```python
from build123d import *

# Parameters (mm, degrees)
SKETCH1_R             = 95
BOSS_EXTRUDE1_DEPTH   = 6
SKETCH2_W             = 55
SKETCH2_H             = 30
CUT_EXTRUDE1_DEPTH    = 135.484199815
CAVITY1_START         = -69.821849164
CAVITY1_OUTLINE_W     = 15
CAVITY1_OUTLINE_H     = 6
CAVITY1_OUTLINE_W_2   = 11
CAVITY1_DEPTH         = 6
CAVITY1_START_2       = 63.821772898
CAVITY1_2_OUTLINE_W   = 11
CAVITY1_2_OUTLINE_H   = 6
CAVITY1_2_OUTLINE_W_2 = 15
CAVITY1_2_DEPTH       = 6
CAVITY1_START_3       = -7.051829773
CAVITY1_3_OUTLINE_W   = 6
CAVITY1_3_OUTLINE_H   = 6
CAVITY1_3_DEPTH       = 14.103659546
CAVITY1_START_4       = -35.551829773
CAVITY1_4_OUTLINE_W   = 6
CAVITY1_4_OUTLINE_H   = 6
CAVITY1_4_DEPTH       = 10.103659546
CAVITY1_START_5       = 25.448170227
CAVITY1_5_OUTLINE_W   = 6
CAVITY1_5_OUTLINE_H   = 6
CAVITY1_5_DEPTH       = 10.103659546
CAVITY1_START_6       = -36.448170227
CAVITY1_6_OUTLINE_W   = 6
CAVITY1_6_OUTLINE_H   = 6
CAVITY1_6_DEPTH       = 0.896340454
CAVITY1_START_7       = -25.448170227
CAVITY1_7_OUTLINE_W   = 6
CAVITY1_7_OUTLINE_H   = 6
CAVITY1_7_DEPTH       = 0.896340454
CAVITY1_START_8       = -7.948170227
CAVITY1_8_OUTLINE_W   = 6
CAVITY1_8_OUTLINE_H   = 6
CAVITY1_8_DEPTH       = 0.896340454
CAVITY1_START_9       = 7.051829773
CAVITY1_9_OUTLINE_W   = 6
CAVITY1_9_OUTLINE_H   = 6
CAVITY1_9_DEPTH       = 0.896340454
CAVITY1_START_10      = 24.551829773
CAVITY1_10_OUTLINE_W  = 6
CAVITY1_10_OUTLINE_H  = 6
CAVITY1_10_DEPTH      = 0.896340454
CAVITY1_START_11      = 35.551829773
CAVITY1_11_OUTLINE_W  = 6
CAVITY1_11_OUTLINE_H  = 6
CAVITY1_11_DEPTH      = 0.896340454
SKETCH3_R             = 1.5
CUT_EXTRUDE3_DEPTH    = 10
CUT_EXTRUDE4_DEPTH    = 135.484199815
CAVITY2_START         = 73.692998072
CAVITY2_OUTLINE_W     = 6
CAVITY2_OUTLINE_H     = 6
CAVITY2_DEPTH         = 6
CUT_EXTRUDE5_DEPTH    = 135.484199815


# Read off the part's stored shape, not the designer's step: Cavity1, Cavity2
with BuildPart() as part:
    # Sketch1 → Boss-Extrude1 (new body)
    with BuildSketch(Plane(origin=(0, 0, 0), x_dir=(1, 0, 0), z_dir=(0, 1, 0))):
        with Locations(Location((0, 0, 0), (0, 0, 270))):
            Circle(SKETCH1_R)
        with BuildLine():
            Line((-36.657195747, -47.5), (36.657195747, -47.5))
            ThreePointArc((36.657195747, -47.5), (0, -60), (-36.657195747, -47.5))
        make_face(mode=Mode.SUBTRACT)
        with BuildLine():
            Line((-42.5, 42.352685865), (-42.5, -42.352685865))
            ThreePointArc((-42.5, -42.352685865), (-60, 0), (-42.5, 42.352685865))
        make_face(mode=Mode.SUBTRACT)
        with BuildLine():
            Line((36.657195747, 47.5), (-36.657195747, 47.5))
            ThreePointArc((-36.657195747, 47.5), (0, 60), (36.657195747, 47.5))
        make_face(mode=Mode.SUBTRACT)
        with BuildLine():
            Line((42.5, -42.352685865), (42.5, 42.352685865))
            ThreePointArc((42.5, 42.352685865), (60, 0), (42.5, -42.352685865))
        make_face(mode=Mode.SUBTRACT)
    extrude(amount=BOSS_EXTRUDE1_DEPTH)

    # Sketch2 → Cut-Extrude1 (cut, through all)
    with BuildSketch(Plane(origin=(0, 6, 0), x_dir=(1, 0, 0), z_dir=(0, 1, 0))):
        Rectangle(SKETCH2_W, SKETCH2_H)
    extrude(amount=-CUT_EXTRUDE1_DEPTH, mode=Mode.SUBTRACT)

    # Cavity1 outline → Cavity1 (cut)
    with BuildSketch(Plane(origin=(0, 0, 0), x_dir=(0.9999872892756082, 0, 0.005041952719030872), z_dir=(0.005041952719030872, 0, -0.9999872892756083)).offset(CAVITY1_START)):
        with Locations((0.448170227, -3)):
            Rectangle(CAVITY1_OUTLINE_W, CAVITY1_OUTLINE_H)
        with Locations((30.948170227, -3)):
            Rectangle(CAVITY1_OUTLINE_W_2, CAVITY1_OUTLINE_H)
        with Locations((-30.051829773, -3)):
            Rectangle(CAVITY1_OUTLINE_W_2, CAVITY1_OUTLINE_H)
    extrude(amount=CAVITY1_DEPTH, mode=Mode.SUBTRACT)

    # Cavity1 2 outline → Cavity1 2 (cut)
    with BuildSketch(Plane(origin=(0, 0, 0), x_dir=(0.9999872892756082, 0, 0.005041952719030872), z_dir=(0.005041952719030872, 0, -0.9999872892756083)).offset(CAVITY1_START_2)):
        with Locations((30.051829773, -3)):
            Rectangle(CAVITY1_2_OUTLINE_W, CAVITY1_2_OUTLINE_H)
        with Locations((-0.448170227, -3)):
            Rectangle(CAVITY1_2_OUTLINE_W_2, CAVITY1_2_OUTLINE_H)
        with Locations((-30.948170227, -3)):
            Rectangle(CAVITY1_2_OUTLINE_W, CAVITY1_2_OUTLINE_H)
    extrude(amount=CAVITY1_2_DEPTH, mode=Mode.SUBTRACT)

    # Cavity1 3 outline → Cavity1 3 (cut)
    with BuildSketch(Plane(origin=(0, 0, 0), x_dir=(0.9999872892756082, 0, 0.005041952719030872), z_dir=(0.005041952719030872, 0, -0.9999872892756083)).offset(CAVITY1_START_3)):
        with Locations((66.821849164, -3)):
            Rectangle(CAVITY1_3_OUTLINE_W, CAVITY1_3_OUTLINE_H)
        with Locations((-66.821849164, -3)):
            Rectangle(CAVITY1_3_OUTLINE_W, CAVITY1_3_OUTLINE_H)
    extrude(amount=CAVITY1_3_DEPTH, mode=Mode.SUBTRACT)

    # Cavity1 4 outline → Cavity1 4 (cut)
    with BuildSketch(Plane(origin=(0, 0, 0), x_dir=(0.9999872892756082, 0, 0.005041952719030872), z_dir=(0.005041952719030872, 0, -0.9999872892756083)).offset(CAVITY1_START_4)):
        with Locations((66.821849164, -3)):
            Rectangle(CAVITY1_4_OUTLINE_W, CAVITY1_4_OUTLINE_H)
        with Locations((-66.821849164, -3)):
            Rectangle(CAVITY1_4_OUTLINE_W, CAVITY1_4_OUTLINE_H)
    extrude(amount=CAVITY1_4_DEPTH, mode=Mode.SUBTRACT)

    # Cavity1 5 outline → Cavity1 5 (cut)
    with BuildSketch(Plane(origin=(0, 0, 0), x_dir=(0.9999872892756082, 0, 0.005041952719030872), z_dir=(0.005041952719030872, 0, -0.9999872892756083)).offset(CAVITY1_START_5)):
        with Locations((66.821849164, -3)):
            Rectangle(CAVITY1_5_OUTLINE_W, CAVITY1_5_OUTLINE_H)
        with Locations((-66.821849164, -3)):
            Rectangle(CAVITY1_5_OUTLINE_W, CAVITY1_5_OUTLINE_H)
    extrude(amount=CAVITY1_5_DEPTH, mode=Mode.SUBTRACT)

    # Cavity1 6 outline → Cavity1 6 (cut)
    with BuildSketch(Plane(origin=(0, 0, 0), x_dir=(0.9999872892756082, 0, 0.005041952719030872), z_dir=(0.005041952719030872, 0, -0.9999872892756083)).offset(CAVITY1_START_6)):
        with Locations((-66.821849164, -3)):
            Rectangle(CAVITY1_6_OUTLINE_W, CAVITY1_6_OUTLINE_H)
    extrude(amount=CAVITY1_6_DEPTH, mode=Mode.SUBTRACT)

    # Cavity1 7 outline → Cavity1 7 (cut)
    with BuildSketch(Plane(origin=(0, 0, 0), x_dir=(0.9999872892756082, 0, 0.005041952719030872), z_dir=(0.005041952719030872, 0, -0.9999872892756083)).offset(CAVITY1_START_7)):
        with Locations((66.821849164, -3)):
            Rectangle(CAVITY1_7_OUTLINE_W, CAVITY1_7_OUTLINE_H)
    extrude(amount=CAVITY1_7_DEPTH, mode=Mode.SUBTRACT)

    # Cavity1 8 outline → Cavity1 8 (cut)
    with BuildSketch(Plane(origin=(0, 0, 0), x_dir=(0.9999872892756082, 0, 0.005041952719030872), z_dir=(0.005041952719030872, 0, -0.9999872892756083)).offset(CAVITY1_START_8)):
        with Locations((-66.821849164, -3)):
            Rectangle(CAVITY1_8_OUTLINE_W, CAVITY1_8_OUTLINE_H)
    extrude(amount=CAVITY1_8_DEPTH, mode=Mode.SUBTRACT)

    # Cavity1 9 outline → Cavity1 9 (cut)
    with BuildSketch(Plane(origin=(0, 0, 0), x_dir=(0.9999872892756082, 0, 0.005041952719030872), z_dir=(0.005041952719030872, 0, -0.9999872892756083)).offset(CAVITY1_START_9)):
        with Locations((66.821849164, -3)):
            Rectangle(CAVITY1_9_OUTLINE_W, CAVITY1_9_OUTLINE_H)
    extrude(amount=CAVITY1_9_DEPTH, mode=Mode.SUBTRACT)

    # Cavity1 10 outline → Cavity1 10 (cut)
    with BuildSketch(Plane(origin=(0, 0, 0), x_dir=(0.9999872892756082, 0, 0.005041952719030872), z_dir=(0.005041952719030872, 0, -0.9999872892756083)).offset(CAVITY1_START_10)):
        with Locations((-66.821849164, -3)):
            Rectangle(CAVITY1_10_OUTLINE_W, CAVITY1_10_OUTLINE_H)
    extrude(amount=CAVITY1_10_DEPTH, mode=Mode.SUBTRACT)

    # Cavity1 11 outline → Cavity1 11 (cut)
    with BuildSketch(Plane(origin=(0, 0, 0), x_dir=(0.9999872892756082, 0, 0.005041952719030872), z_dir=(0.005041952719030872, 0, -0.9999872892756083)).offset(CAVITY1_START_11)):
        with Locations((66.821849164, -3)):
            Rectangle(CAVITY1_11_OUTLINE_W, CAVITY1_11_OUTLINE_H)
    extrude(amount=CAVITY1_11_DEPTH, mode=Mode.SUBTRACT)

    # Sketch3 → Cut-Extrude3 (cut)
    with BuildSketch(Plane(origin=(0, 6, 0), x_dir=(1, 0, 0), z_dir=(0, 1, 0))):
        with Locations(Location((-31.04, -34.8, 0), (0, 0, 270))):
            Circle(SKETCH3_R)
        with Locations(Location((-31.04, 34.6, 0), (0, 0, 270))):
            Circle(SKETCH3_R)
        with Locations(Location((36.78, -11.31, 0), (0, 0, 270))):
            Circle(SKETCH3_R)
        with BuildLine():
            ThreePointArc((36.657195747, -18.81), (29.157195747, -11.31), (36.657195747, -3.81))
            Line((36.657195747, -3.81), (36.657195747, 34.6))
            Line((36.657195747, 34.6), (-23.54, 34.6))
            ThreePointArc((-23.54, 34.6), (-25.736699141, 29.296699141), (-31.04, 27.1))
            Line((-31.04, 27.1), (-31.04, -27.3))
            ThreePointArc((-31.04, -27.3), (-25.736699141, -29.496699141), (-23.54, -34.8))
            Line((-23.54, -34.8), (36.657195747, -34.8))
            Line((36.657195747, -34.8), (36.657195747, -18.81))
        make_face()
    extrude(amount=-CUT_EXTRUDE3_DEPTH, mode=Mode.SUBTRACT)

    # Sketch4 → Cut-Extrude4 (cut, through all)
    with BuildSketch(Plane(origin=(0, 6, 0), x_dir=(1, 0, 0), z_dir=(0, 1, 0))):
        Polygon((39.849101937, -61.771443224), (35.488287493, -57.506083054), (42.620529088, -50.214229392), (46.981343533, -54.479589562), align=None)
        Polygon((53.83388938, -47.473690947), (60.966130976, -40.181837285), (56.605316531, -35.916477115), (49.473074935, -43.208330777), align=None)
        Polygon((-61.771443224, -39.849101937), (-57.506083054, -35.488287493), (-50.214229392, -42.620529088), (-54.479589562, -46.981343533), align=None)
        Polygon((-47.473690947, -53.83388938), (-43.208330777, -49.473074935), (-35.916477115, -56.605316531), (-40.181837285, -60.966130976), align=None)
        Polygon((-39.849101937, 61.771443224), (-35.488287493, 57.506083054), (-42.620529088, 50.214229392), (-46.981343533, 54.479589562), align=None)
        Polygon((-53.83388938, 47.473690947), (-49.473074935, 43.208330777), (-56.605316531, 35.916477115), (-60.966130976, 40.181837285), align=None)
        Polygon((61.771443224, 39.849101937), (57.506083054, 35.488287493), (50.214229392, 42.620529088), (54.479589562, 46.981343533), align=None)
        Polygon((47.473690947, 53.83388938), (43.208330777, 49.473074935), (35.916477115, 56.605316531), (40.181837285, 60.966130976), align=None)
    extrude(amount=-CUT_EXTRUDE4_DEPTH, mode=Mode.SUBTRACT)

    # Cavity2 outline → Cavity2 (cut)
    with BuildSketch(Plane(origin=(0, 0, 0), x_dir=(0, 1, 0), z_dir=(0.9999872892756082, 0, 0.005041952719040901)).offset(CAVITY2_START)):
        with Locations((3, -19.041827)):
            Rectangle(CAVITY2_OUTLINE_W, CAVITY2_OUTLINE_H)
        with Locations((3, 19.958173)):
            Rectangle(CAVITY2_OUTLINE_W, CAVITY2_OUTLINE_H)
    extrude(amount=CAVITY2_DEPTH, mode=Mode.SUBTRACT)

    # Sketch5 → Cut-Extrude5 (cut, through all)
    with BuildSketch(Plane(origin=(0, 6, 0), x_dir=(1, 0, 0), z_dir=(0, 1, 0))):
        Polygon((15.670066484, -73.772943514), (21.66999022, -73.80319523), (21.639738504, -79.803118966), (15.639814768, -79.77286725), align=None)
        Polygon((-23.329437797, -73.576307358), (-23.359689514, -79.576231094), (-17.359765778, -79.60648281), (-17.329514062, -73.606559074), align=None)
        Polygon((-73.772943514, -15.670066484), (-73.80319523, -21.66999022), (-79.803118966, -21.639738504), (-79.77286725, -15.639814768), align=None)
        Polygon((-73.576307358, 23.329437797), (-79.576231094, 23.359689514), (-79.60648281, 17.359765778), (-73.606559074, 17.329514062), align=None)
        Polygon((-15.670066484, 73.772943514), (-21.66999022, 73.80319523), (-21.639738504, 79.803118966), (-15.639814768, 79.77286725), align=None)
        Polygon((23.329437797, 73.576307358), (23.359689514, 79.576231094), (17.359765778, 79.60648281), (17.329514062, 73.606559074), align=None)
    extrude(amount=-CUT_EXTRUDE5_DEPTH, mode=Mode.SUBTRACT)


solid = part.part
```
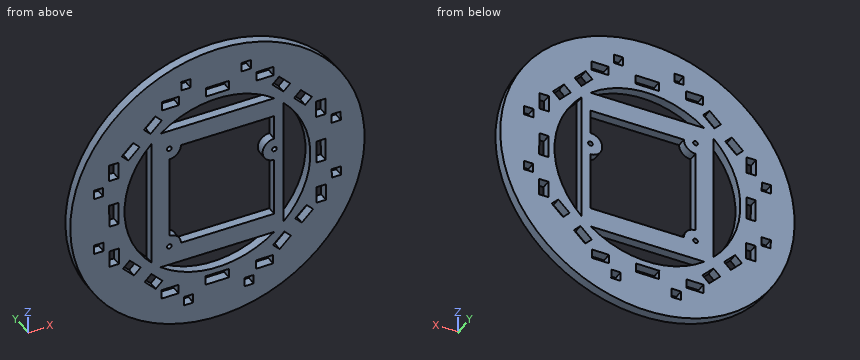
Geometry: final body of the model. Coordinates: model frame, mm. Coordinates: 2 decimals unless noted, no trailing zeros. Loops run counter-clockwise (first coordinate to the right, second up) from the corner with the lowest first, then second, coordinate; pieces in that order, holes last. Notation, with made-up numbers: M 19,89 L 52,89 A25 cw 52,126 Z; hole C 26.25,-1 d7. An arc over 180 degrees is marked long. Put each result on its own line as item: value.
(1) First-contact query: pin 1 (1.5 mm diameter, centred on x = -36.5, y = 2, fed in from +Z); pin 2 (1 mm diameter, centred on y = 3, z = 17.5, fed in from +X); pin 3 (1.5 mm diameter, centred on y = 4.5, z = -9, fed in from -X); pin 4 (2.5 mm diameter, centred on x = 36.78, z = 11.31, fed in from +Y). Flat tips, straight axial feed; report the tip coordinate or a pass-through.
Answer sheet:
pin 1: stops at z = 88.02
pin 2: stops at x = 93.47
pin 3: stops at x = -94.64
pin 4: passes through
(2) Cut plane B-B on y = 1.25. State how many separate pieces and enclosed holes the cut face has, then the cut area to 3 significant figures.
Answer sheet:
separate pieces: 1
enclosed holes: 36
area: 18,800 mm^2
(3) Cut plane A-A on x = 0. Return the cut outline in (y, z), then the cut area to 3 significant figures.
Answer sheet:
outline: M 0,-95 L 6,-95 L 6,-69.82 L 0,-69.82 Z; M 0,-63.82 L 6,-63.82 L 6,-60 L 0,-60 Z; M 0,-47.5 L 6,-47.5 L 6,-34.6 L 0,-34.6 Z; M 0,34.8 L 6,34.8 L 6,47.5 L 0,47.5 Z; M 0,60 L 6,60 L 6,63.82 L 0,63.82 Z; M 0,69.82 L 6,69.82 L 6,95 L 0,95 Z
area: 502 mm^2
(4) Material intervals for probe 1 along X at (y, z) = (1.5, 66.5); probe 2 along X at (y, z) = (3.5, 45); probe 3 along Z at (x, y) = (-13.5, 4), sorted ascending.
Answer sheet:
probe 1: x = -67.84 to -35.89, -24.89 to -7.39, 7.61 to 25.11, 36.11 to 67.84
probe 2: x = -83.67 to -56.51, -52.54 to 51.3, 56.25 to 83.67
probe 3: z = -94.04 to -58.46, -47.5 to -34.6, 34.8 to 47.5, 58.46 to 94.04
(5) Cut plane C-C on x = 83. Return the cut outline in (y, z), then the cut area to 3 significant figures.
Answer sheet:
outline: M 0,-46.22 L 6,-46.22 L 6,46.22 L 0,46.22 Z
area: 555 mm^2
